```python
from build123d import *

# Parameters (mm, degrees)
SKETCH1_W           = 25.4
SKETCH1_H           = 25.4
BOSS_EXTRUDE1_DEPTH = 508


with BuildPart() as part:
    # Sketch1 → Boss-Extrude1 (new body)
    with BuildSketch(Plane(origin=(0, 0, 0), x_dir=(1, 0, 0), z_dir=(0, 1, 0))):
        with Locations((12.7, 12.7)):
            Rectangle(SKETCH1_W, SKETCH1_H)
        Polygon((1.27, 12.361459156), (1.27, 24.13), (12.7, 24.13), (24.13, 24.13), (24.13, 12.7), (24.13, 1.27), (12.7, 1.27), (1.27, 1.27), align=None, mode=Mode.SUBTRACT)
    extrude(amount=BOSS_EXTRUDE1_DEPTH)


solid = part.part
```
The listing builds one solid part. Answer for the finished solid, in the listing's coordinates (mm). A direction names the side the tool comes from. Coordinates: 2 decimals unless noted, no trailing zeros. Loops run counter-clockwise (first coordinate to the right, second up) from the corner with the lowest first, then second, coordinate; pieces in that order, holes last. Notation, with made-up numbers: M 60.5,70 L 113.5,70 A12 ccw 113.5,78 Z; hole C 36,14.5 d6. An arc over 180 degrees is marked long. Answer as a JSON object with one key per item and string values. Group by question number.
Item 1: Section A-A (x = 18.75) is taken. Write down the section's boundary in (y, z), and give its area (3 significant figures).
Item 2: Section B-B (z = -5.5) is taken. Write down the section's boundary in (x, y), and give its area (3 significant figures).
Item 3: Section C-C (y = 334) is taken. Write down the section's boundary in (x, z), and give its area (3 significant figures).
Item 4: Which of the six approach directions +Z, -Z, +X, -X, +Y, -Y give full straight-line access (tool end or side, diameter ignored) to faces 1 (the face through (12, 508, -1)), 2 (the face through (1.27, 250, -13))?
Item 5: Determine the mould class of faces 3 (the face through (24.13, 250, -13)), 4 (the face through (13, 250, -24.13)), 5 (the face through (13, 250, -25.4)), 6 (the face through (12, 0, -1)) for opening direction Z: +Z half, -Z half, draft (parallel to the pull), parting line (faces both ways), or undercut.
Item 6: Consider L1, parallel to Z at x = 3.25, y = 22; L2, parallel to X at y = 107, z = -7. Determine where each line is inside the solid, lowest interval first.
Solved:
{
 "1": {"outline": "M 0,-25.4 L 508,-25.4 L 508,-24.13 L 0,-24.13 Z; M 0,-1.27 L 508,-1.27 L 508,0 L 0,0 Z", "area": "1,290 mm2"},
 "2": {"outline": "M 0,0 L 1.27,0 L 1.27,508 L 0,508 Z; M 24.13,0 L 25.4,0 L 25.4,508 L 24.13,508 Z", "area": "1,290 mm2"},
 "3": {"outline": "M 0,-25.4 L 25.4,-25.4 L 25.4,0 L 0,0 Z; hole M 1.27,-24.13 L 24.13,-24.13 L 24.13,-1.27 L 1.27,-1.27 Z", "area": "123 mm2"},
 "4": {"face 1": "+Z, -Z, +X, -X, +Y", "face 2": "+Y, -Y"},
 "5": {"face 3": "undercut", "face 4": "undercut", "face 5": "-Z half", "face 6": "draft"},
 "6": {"L1": "z = -25.4 to -24.13, -1.27 to 0", "L2": "x = 0 to 1.27, 24.13 to 25.4"}
}
